from build123d import *

# Parameters (mm, degrees)
F0_W     = 1295.4
F0_H     = 38.1
F1_DEPTH = 38.1
F2_W     = 88.9
F2_H     = 361.95
F2_H_2   = 38.1
F3_DEPTH = 19.05


with BuildPart() as f1:
    # F0 (on Top) → F1 (new body)
    with BuildSketch(Plane.XY):
        with Locations((647.7, -342.9)):
            Rectangle(F0_W, F0_H)
    extrude(amount=F1_DEPTH)

    # F2 (on face) → F3 (join)
    with BuildSketch(Plane.XY.offset(38.1)):
        with Locations((647.7, -180.975)):
            Rectangle(F2_W, F2_H)
        with Locations((850.9, -180.975)):
            Rectangle(F2_W, F2_H)
        with Locations((1054.1, -180.975)):
            Rectangle(F2_W, F2_H)
        with Locations((1257.3, -180.975)):
            Rectangle(F2_W, F2_H)
        with Locations((444.5, -180.975)):
            Rectangle(F2_W, F2_H)
        with Locations((241.3, -180.975)):
            Rectangle(F2_W, F2_H)
        with Locations((38.1, -180.975)):
            Rectangle(F2_W, F2_H)
        with Locations((749.3, -342.9)):
            Rectangle(F2_W, F2_H_2)
        with Locations((952.5, -342.9)):
            Rectangle(F2_W, F2_H_2)
        with Locations((1155.7, -342.9)):
            Rectangle(F2_W, F2_H_2)
        with Locations((546.1, -342.9)):
            Rectangle(F2_W, F2_H_2)
        with Locations((342.9, -342.9)):
            Rectangle(F2_W, F2_H_2)
        with Locations((139.7, -342.9)):
            Rectangle(F2_W, F2_H_2)
    extrude(amount=F3_DEPTH)

    # F4: F1 across plane


with BuildPart() as f1_1:
    add(f1.part)
    add(f1.part.mirror(Plane.XZ))


solid = f1_1.part
Design review of the part built by this model. Coordinates are the model's own, in mm. A direction names the side the tool comes from. Round coordinates to 2 decimals unless told otherwise and drop trailing zeros. Loops run counter-clockwise (first coordinate to the right, second up) from the corner with the lowest first, then second, coordinate; pieces in that order, holes last. Notation, with made-up numbers: (24, 33) - (48, 33) arc R29 ccw to (48, 56) - close; hole circle Ø2 at (85.25, -18). An arc over 180 degrees is marked (long way). One line per question, with ' | ' between items.
1. Draft analysis for pull direction Y (two halves, no side actions). For faces 4 (the face through (639, 361.95, 28)), 5 (the face through (647, -5, 57.15)), 6 (the face through (639, -323.85, 22)), state which applies: released by +Y, released by -Y, zero draft, split by the parting line, or undercut.
Results are:
face 4: released by +Y | face 5: zero draft | face 6: undercut
2. We need section C-C, the plane z = 27. State the section outline as (x, y) points, and give its area (3 significant figures).
Results are:
outline: (0, -361.95) - (1295.4, -361.95) - (1295.4, -323.85) - (0, -323.85) - close; (0, 323.85) - (1295.4, 323.85) - (1295.4, 361.95) - (0, 361.95) - close | area: 98,700 mm²
3. For faces 1 (the face through (647, -5, 38.1)), 2 (the face through (342, 343, 57.15)), 3 (the face through (1295.4, 343, 19)), list the 3-axis set-ups (+Z, -Z, +X, -X, +Y, -Y) from which the entire face can be reached by the end or side of a thin tool; tool diameter is ignored.
Results are:
face 1: -Z, +X, -X | face 2: +Z, +X, -X, +Y, -Y | face 3: -Z, +X, +Y, -Y
4. We need section A-A, the plane y = 221.5. State the section outline as (x, z) points.
Results are:
outline: (-6.35, 38.1) - (82.55, 38.1) - (82.55, 57.15) - (-6.35, 57.15) - close; (196.85, 38.1) - (285.75, 38.1) - (285.75, 57.15) - (196.85, 57.15) - close; (400.05, 38.1) - (488.95, 38.1) - (488.95, 57.15) - (400.05, 57.15) - close; (603.25, 38.1) - (692.15, 38.1) - (692.15, 57.15) - (603.25, 57.15) - close; (806.45, 38.1) - (895.35, 38.1) - (895.35, 57.15) - (806.45, 57.15) - close; (1009.65, 38.1) - (1098.55, 38.1) - (1098.55, 57.15) - (1009.65, 57.15) - close; (1212.85, 38.1) - (1301.75, 38.1) - (1301.75, 57.15) - (1212.85, 57.15) - close
5. We need section B-B, the plane x = 368. State the section outline as (y, z) points, and give its area (3 significant figures).
Results are:
outline: (-361.95, 0) - (-323.85, 0) - (-323.85, 57.15) - (-361.95, 57.15) - close; (323.85, 0) - (361.95, 0) - (361.95, 57.15) - (323.85, 57.15) - close | area: 4,350 mm²
6. We need section D-D, the plane x = 878. State the section outline as (y, z) points.
Results are:
outline: (-361.95, 0) - (-323.85, 0) - (-323.85, 38.1) - (323.85, 38.1) - (323.85, 0) - (361.95, 0) - (361.95, 57.15) - (-361.95, 57.15) - close
7. Clearance check with flat-ended pins moving along their axes: P1, Ø10, axis at x = 1000, y = -349, coming from the +Z side; P2, Ø6.5, axis at x = 697, y = 348.5, coming from the +Z side. State where each tip first meets the part, or that it passes through.
Results are:
P1: stops at z = 57.15 | P2: stops at z = 38.1
8. For L1, parallel to Y at x = 1050, z = 38; L2, parallel to Z at x = 472.5, y = -156; L3, parallel to X at y = 330, z = 13, list the stretches that pass through material, from the lowest coordinate up. Write a range as [from, to].
Results are:
L1: y = [-361.95, -323.85], [323.85, 361.95] | L2: z = [38.1, 57.15] | L3: x = [0, 1295.4]
